from build123d import *

# Parameters (mm, degrees)
CROQUIS1_W              = 52.8
CROQUIS1_H              = 40.9
SALIENTE_EXTRUIR1_DEPTH = 2.5
CORTAR_EXTRUIR1_DEPTH   = 44
CROQUIS3_R              = 1.25
CORTAR_EXTRUIR2_DEPTH   = 44


with BuildPart() as part:
    # Croquis1 → Saliente-Extruir1 (new body)
    with BuildSketch(Plane(origin=(0, 0, 0), x_dir=(1, 0, 0), z_dir=(0, 1, 0))):
        with Locations((7.799477352, -11.379703833)):
            Rectangle(CROQUIS1_W, CROQUIS1_H)
    extrude(amount=SALIENTE_EXTRUIR1_DEPTH)

    # Croquis2 → Cortar-Extruir1 (cut)
    with BuildSketch(Plane.XY.offset(31.829703833)):
        with BuildLine():
            Line((-18.600522648, 2.5), (34.199477352, 2.5))
            ThreePointArc((34.199477352, 2.5), (7.799477352, 1.421940601), (-18.600522648, 2.5))
        make_face()
    extrude(amount=-CORTAR_EXTRUIR1_DEPTH, mode=Mode.SUBTRACT)

    # Croquis3 → Cortar-Extruir2 (cut)
    with BuildSketch(Plane.XZ):
        with Locations((23.949477352, 11.379703833)):
            Circle(CROQUIS3_R)
        with Locations((-8.350522648, 11.379703833)):
            Circle(CROQUIS3_R)
    extrude(amount=-CORTAR_EXTRUIR2_DEPTH, mode=Mode.SUBTRACT)


solid = part.part
Geometry check sheet. Reference: the model listing, model coordinates, mm. Round coordinates to 2 decimals unless told otherwise and drop trailing zeros. Write each loop counter-clockwise with the first axis right and the second up, starting at its lowest first coordinate (ties: lowest second). Pieces come first, ordered by that corner, then holes.
Item 1: Material ranges on line 1 along Z through (x, y) = (-9, 0.85); line 2 along Y through (x, z) = (2, 1); line 3 along Y through (x, z) = (-4, 26.5), recorded low to high.
Determined:
line 1: z = -9.07 to 10.31, 12.45 to 31.83
line 2: y = 0 to 1.47
line 3: y = 0 to 1.64
Item 2: Section check B-B (z = 9). Record the boundary of the cut face in (x, y), plus the area to 3 significant figures.
Determined:
outline: (-18.6, 0) - (34.2, 0) - (34.2, 2.5) arc R323.79 cw to (-18.6, 2.5) - close
area: 94.0 mm2
Item 3: Section check C-C (x = -14). Record the boundary of the cut face in (y, z).
Determined:
outline: (0, -9.07) - (2.16, -9.07) - (2.16, 31.83) - (0, 31.83) - close
Item 4: Mould release check, pull along X, two halves, no side actions. Record for faces 1 (the face through (-18.601, 1, 12)), 2 (the face through (7, 0, 11)), 3 (the face through (25.104, 0.932, 10.901)): +X half, -X half, draft (parallel to the pull), parting line (faces both ways), or undercut.
Determined:
face 1: -X half
face 2: draft
face 3: undercut
Item 5: Section check A-A (x = -8). Record the boundary of the cut face in (y, z).
Determined:
outline: (0, -9.07) - (1.81, -9.07) - (1.81, 10.18) - (0, 10.18) - close; (0, 12.58) - (1.81, 12.58) - (1.81, 31.83) - (0, 31.83) - close
Item 6: Go/stop test with flat-tipped pins: pin 1 Ø2 at (x, z) = (-8.35, 11.38) entering from +Y; pin 2 Ø4 at (x, z) = (-12.5, 4.5) entering from +Y. Record where each tip stops, or that it passes through.
Determined:
pin 1: passes through
pin 2: stops at y = 2.19
